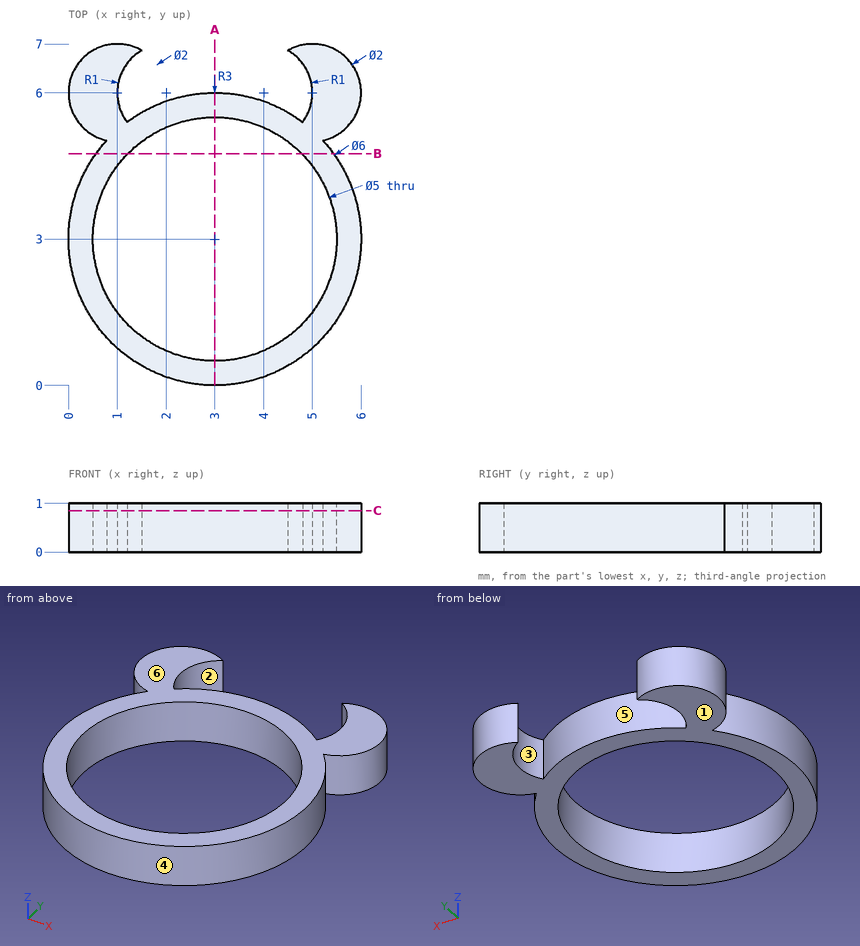
Source: three-view drawing plus pictorial views. Frame: mm from the lowest corner of the part. A direction names the side the tool comes from. Give positions to 0.01 mm unless a question says otherwise; leave off trailing zeros. Order: outer loops, then holes, each group sorted by start corner. A loop starts at its lowest first (then second) coordinate and runs counter-clockwise, first axis right, second up. Notation, with made-up numbers: (-33, 58.5) -> (-16, 58.5) arc R12 ccw to (-16, 79.5) -> close; hole circle Ø4 at (34, -40). An arc over 180 degrees is marked (long way). Put each result on its own line as item: value.
Q1. Section C-C, the plane z = 0.85. Return loops of the section in (x, y).
Here are the results:
outline: (0.79, 5.02) arc R3 ccw (long way) to (5.21, 5.02) arc R1 ccw (long way) to (4.5, 6.87) arc R1 cw to (4.8, 5.4) arc R3 ccw to (1.2, 5.4) arc R1 cw to (1.5, 6.87) arc R1 ccw (long way) to start; hole circle Ø5 at (3, 3)
Q2. Section B-B, the plane y = 4.75. Return loops of the section in (x, z), then the cut area to 3 significant figures.
Here are the results:
outline: (0.56, 0) -> (1.21, 0) -> (1.21, 1) -> (0.56, 1) -> close; (4.79, 0) -> (5.44, 0) -> (5.44, 1) -> (4.79, 1) -> close
area: 1.30 mm^2
Q3. Reachability of the marked faces 5 and 6 from +Z, -Z, +X, -X, +Y, -Y: full face, straight path, thin tool, end or side. Return the list, or none.
Here are the results:
face 5: +Z, -Z
face 6: +Z, +X, -X, +Y, -Y
Q4. Section A-A, the plane x = 3. Return loops of the section in (y, z).
Here are the results:
outline: (0, 0) -> (0.5, 0) -> (0.5, 1) -> (0, 1) -> close; (5.5, 0) -> (6, 0) -> (6, 1) -> (5.5, 1) -> close
Q5. Material intervals for L1, parallel to Y at x = 3, z = 0.3; L2, parallel to X at y = 1.75, z = 0.5; L3, parallel to Y at x = 2, z = 0.8, sorted ascending.
Here are the results:
L1: y = 0 to 0.5, 5.5 to 6
L2: x = 0.27 to 0.83, 5.17 to 5.73
L3: y = 0.17 to 0.71, 5.29 to 5.83
Q6. Draft query along X for the marked faces 1, 2, 3 and 4. Return one class per face: released by +X, released by -X, zero draft, split by the parting line, or undercut.
Here are the results:
face 1: zero draft
face 2: undercut
face 3: undercut
face 4: split by the parting line
